Autodesk Inventor part; units mm, degrees
ref_plane "YZ Plane" through (0, 0, 0) normal (1, 0, 0) x (0, 1, 0)
ref_plane "XZ Plane" through (0, 0, 0) normal (0, 1, 0) x (-1, 0, 0)
ref_plane "XY Plane" through (0, 0, 0) normal (0, 0, 1) x (1, 0, 0)
sketch "Skizze8" plane through (0, 0, 0) normal (0, 0, 1) x (1, 0, 0)
  line L0 (-10, -5) -> (10, -5)
  line L1 (10, -5) -> (10, 5)
  line L2 (10, 5) -> (-10, 5)
  line L3 (-10, 5) -> (-10, -5)
  line L4 (-10, -5) -> (10, 5) construction
  line L5 (10, -5) -> (-10, 5) construction
  point P0 (0, 0)
  dimension "d49" = 10
  dimension "d50" = 20
extrude "Grundkörper" add sketch "Skizze8" along normal blind 100
sketch "Skizze9" plane through (-10, -5, 0) normal (0, -1, 0) x (1, 0, 0)
  line L0 (10, 120) -> (10, -20) construction
  line L1 (0, 0) -> (20, 0) construction
  point P0 (10, 0)
  point P1 (10, 9)
  point P2 (10, 38.5)
  dimension "d53" = 9
  dimension "d54" = 38.5
hole "DIN7984_M5" at (0, -5, 9) at (0, -5, 38.5) direction (0, 1, 0) diameter 5.5 end through all counterbore diameter 10 counterbore depth 3.9
sketch "Skizze10" plane through (-10, 5, 0) normal (0, 1, 0) x (1, 0, 0)
  line L0 (10, 20) -> (10, -120) construction
  line L1 (20, -100) -> (0, -100)
  point P0 (10, 0)
  point P1 (10, -92)
  dimension "d62" = 8
hole "M6" at (0, 5, 92) direction (0, -1, 0) diameter 4.917 end through all countersink diameter 6 countersink angle 90
chamfer "Fase_Abschraegung" distance 5 angle 45 2 edges at (-10, 0, 100) (10, 0, 100)
chamfer "Fase_Allgemein" distance 1 angle 45 10 edges at (-10, -5, 47.5) (-7.5, -5, 97.5) (0, -5, 100) (7.5, -5, 97.5) (10, -5, 47.5) (-10, 5, 47.5) (-7.5, 5, 97.5) (0, 5, 100) (7.5, 5, 97.5) (10, 5, 47.5)
properties part number "200-60-DIFFERENTIAL-BAR-01" material "Aluminium 6061"
Design review of the part built by this model. Coordinates are the model's own, in mm. A direction names the side the tool comes from. Round coordinates to 2 decimals unless told otherwise and drop trailing zeros. Order: outer loops, then holes, each group sorted by start corner. A loop starts at its lowest first (then second) coordinate and runs counter-clockwise, first axis right, second up. Notation, with made-up numbers: (64, -3) - (117, -3) arc R23 cw to (117, 36) - close; hole circle Ø5 at (67.25, 65). An arc over 180 degrees is marked (long way). One line per question, with ' | ' between items.
Item 1: Wall thickness on line 1 (Z direction, x = 0, y = 1.25); line 2 (Z direction, x = 0, y = -2.2); line 3 (X direction, y = 0.5, z = 38.5): over which ranges is each line inside the solid? List them lowest first. Write a range as [from, to].
Checks:
line 1: [0, 6.25], [11.75, 35.75], [41.25, 89.54], [94.46, 100] | line 2: [0, 4], [14, 33.5], [43.5, 89.54], [94.46, 100] | line 3: [-10, -2.75], [2.75, 10]
Item 2: For P1, Ø3, axis at x = 1, z = 36.5, coming from the -Y side, flat-tipped, find the tip position at first contact; note if it passes through.
Checks:
P1: y = -1.1
Item 3: Take a section at A-A, the plane z = 92. Write out the cut boundary in (x, y).
Checks:
outline: (-10, -4) - (-9, -5) - (-2.46, -5) - (-2.46, 4.46) - (-3, 5) - (-9, 5) - (-10, 4) - close; (2.46, -5) - (9, -5) - (10, -4) - (10, 4) - (9, 5) - (3, 5) - (2.46, 4.46) - close
Item 4: Take a section at B-B, the plane x = 0. Write out the cut boundary in (y, z), then the cut area to 3 significant figures.
Checks:
outline: (-5, 0) - (5, 0) - (5, 6.25) - (-1.1, 6.25) - (-1.1, 4) - (-5, 4) - close; (-5, 14) - (-1.1, 14) - (-1.1, 11.75) - (5, 11.75) - (5, 35.75) - (-1.1, 35.75) - (-1.1, 33.5) - (-5, 33.5) - close; (-5, 43.5) - (-1.1, 43.5) - (-1.1, 41.25) - (5, 41.25) - (5, 89) - (4.46, 89.54) - (-5, 89.54) - close; (-5, 94.46) - (4.46, 94.46) - (5, 95) - (5, 99) - (4, 100) - (-4, 100) - (-5, 99) - close | area: 804 mm²
Item 5: Take a section at D-D, the plane z = 9. Write out the cut boundary in (x, y), then the cut area to 3 significant figures.
Checks:
outline: (-10, -4) - (-9, -5) - (-5, -5) - (-5, -1.1) - (-2.75, -1.1) - (-2.75, 5) - (-9, 5) - (-10, 4) - close; (2.75, -1.1) - (5, -1.1) - (5, -5) - (9, -5) - (10, -4) - (10, 4) - (9, 5) - (2.75, 5) - close | area: 125 mm²
Item 6: Draft analysis for pull direction X (two halves, no side actions). For faces 3 (the face through (-10, 0, 47)), 4 (the face through (0, 0, 0)), 5 (the face through (-0.22, -3.023, 43.495)), state which applies: +X half, -X half, draft (parallel to the pull), parting line (faces both ways), or undercut.
Checks:
face 3: -X half | face 4: draft | face 5: undercut
Item 7: Machinability: for faces 1 (the face through (8, 0, 97)), 2 (the face through (2, -1.1, 36)), which of the approach directions +Z, -Z, +X, -X, +Y, -Y give a long, thin tool a straight path to every point of the face, cutting with its end or side? Answer none if there is none.
Checks:
face 1: +Z, +X, +Y, -Y | face 2: -Y
Item 8: Take a section at C-C, the plane y = -2.5. Write out the cut boundary in (x, z), then the cut area to 3 significant figures.
Checks:
outline: (-10, 0) - (10, 0) - (10, 95) - (5, 100) - (-5, 100) - (-10, 95) - close; hole circle Ø10 at (0, 9); hole circle Ø10 at (0, 38.5); hole circle Ø4.92 at (0, 92) | area: 1,800 mm²
